Read the model definition and answer for the solid it produces. Units are mm, in the model's axes. Face numbers are marked on the shaded views. Coordinates: 2 decimals unless noted, no trailing zeros. Write each loop counter-clockwise with the first axis right and the second up, starting at its lowest first coordinate (ties: lowest second). Pieces come first, ordered by that corner, then holes. Notation, with made-up numbers: (26.25, 52.25) - (66.25, 52.25) arc R25 cw to (66.25, 77.25) - close; hole circle Ø1 at (-2.5, 59.25). An arc over 180 degrees is marked (long way). Return JSON: item names as keys, results as strings.
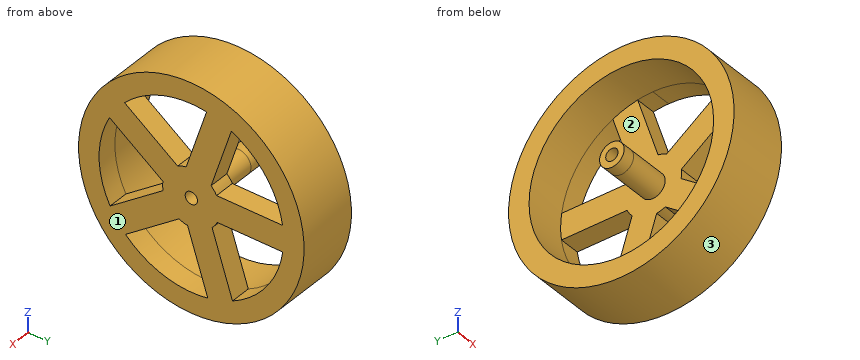
```python
from build123d import *

# Parameters (mm, degrees)
SKETCH1_R           = 27.5
BOSS_EXTRUDE1_DEPTH = 15
SKETCH2_R           = 1.5
CUT_EXTRUDE1_DEPTH  = 16
SKETCH3_R           = 22.5
SKETCH3_R_2         = 3
CUT_EXTRUDE2_DEPTH  = 10
SKETCH4_R           = 3
SKETCH4_R_2         = 1.5
BOSS_EXTRUDE2_DEPTH = 3
CUT_EXTRUDE3_DEPTH  = 6


with BuildPart() as part:
    # Sketch1 → Boss-Extrude1 (new body)
    with BuildSketch(Plane(origin=(0, 0, 0), x_dir=(0, 0, -1), z_dir=(1, 0, 0))):
        Circle(SKETCH1_R)
    extrude(amount=BOSS_EXTRUDE1_DEPTH)

    # Sketch2 → Cut-Extrude1 (cut, through all)
    with BuildSketch(Plane(origin=(15, 0, 0), x_dir=(0, 0, -1), z_dir=(1, 0, 0))):
        Circle(SKETCH2_R)
    extrude(amount=-CUT_EXTRUDE1_DEPTH, mode=Mode.SUBTRACT)

    # Sketch3 → Cut-Extrude2 (cut)
    with BuildSketch(Plane.ZY):
        Circle(SKETCH3_R)
        Circle(SKETCH3_R_2, mode=Mode.SUBTRACT)
    extrude(amount=-CUT_EXTRUDE2_DEPTH, mode=Mode.SUBTRACT)

    # Sketch4 → Boss-Extrude2 (add)
    with BuildSketch(Plane.ZY):
        Circle(SKETCH4_R)
        Circle(SKETCH4_R_2, mode=Mode.SUBTRACT)
    extrude(amount=BOSS_EXTRUDE2_DEPTH)

    # Sketch5 → Cut-Extrude3 (cut, through all)
    with BuildSketch(Plane.ZY.offset(-10)):
        with BuildLine():
            Line((5.074237821, 4.822044228), (20.272779151, 9.76034966))
            ThreePointArc((20.272779151, 9.76034966), (13.350301343, 18.111307353), (3.325036991, 22.252957759))
            Line((3.325036991, 22.252957759), (3.325036991, 6.1598806))
            ThreePointArc((3.325036991, 6.1598806), (4.252576382, 5.560179324), (5.074237821, 4.822044228))
        make_face()
        with BuildLine():
            Line((-3.018010865, 6.315980559), (-3.018010865, 22.296672631))
            ThreePointArc((-3.018010865, 22.296672631), (-13.099406882, 18.293592849), (-20.136327546, 10.03884022))
            Line((-20.136327546, 10.03884022), (-4.830901647, 5.065805886))
            ThreePointArc((-4.830901647, 5.065805886), (-3.973926406, 5.762630382), (-3.018010865, 6.315980559))
        make_face()
        with BuildLine():
            Line((-6.939471114, -0.91855357), (-22.138012444, 4.019751862))
            ThreePointArc((-22.138012444, 4.019751862), (-21.446180029, -6.805245196), (-15.769971823, -16.048613295))
            Line((-15.769971823, -16.048613295), (-6.310698406, -3.029040382))
            ThreePointArc((-6.310698406, -3.029040382), (-6.70859797, -1.998677884), (-6.939471114, -0.91855357))
        make_face()
        with BuildLine():
            Line((10.389948957, -19.957428709), (0.93067554, -6.937855796))
            ThreePointArc((0.93067554, -6.937855796), (-0.172215156, -6.997881246), (-1.270818148, -6.883677886))
            Line((-1.270818148, -6.883677886), (-10.664033269, -19.812329354))
            ThreePointArc((-10.664033269, -19.812329354), (-0.155061304, -22.499465682), (10.389948957, -19.957428709))
        make_face()
        with BuildLine():
            ThreePointArc((22.5, 0), (22.422695556, 1.863524623), (22.19131342, 3.714244025))
            Line((22.19131342, 3.714244025), (6.885887521, -1.258790309))
            ThreePointArc((6.885887521, -1.258790309), (6.60216315, -2.326250576), (6.154062305, -3.335793331))
            Line((6.154062305, -3.335793331), (15.547277427, -16.264444799))
            ThreePointArc((15.547277427, -16.264444799), (20.688931124, -8.844101365), (22.5, 0))
        make_face()
    extrude(amount=-CUT_EXTRUDE3_DEPTH, mode=Mode.SUBTRACT)


solid = part.part
```
(1) Straight lines are drawn through the part: line 1 (Y direction, x = 8.75, z = 0); line 2 (Y direction, x = 11, z = 0); line 3 (Y direction, x = -2.1, z = 0). For each, find the intervals that lie inside material, in ascending order. Write a range as from..to.
Answer:
{"line 1": "-27.5..-22.5, -3..-1.5, 1.5..3, 22.5..27.5", "line 2": "-27.5..-22.5, -7..-1.5, 1.5..27.5", "line 3": "-3..-1.5, 1.5..3"}
(2) A cutting plane is placed at A-A (z = 0). Determine the outline of the cut face in (x, y), and give its area (4 significant figures).
Answer:
{"outline": "(-3, -3) - (10, -3) - (10, -7) - (15, -7) - (15, -1.5) - (-3, -1.5) - close; (-3, 1.5) - (15, 1.5) - (15, 27.5) - (0, 27.5) - (0, 22.5) - (10, 22.5) - (10, 3) - (-3, 3) - close; (0, -27.5) - (15, -27.5) - (15, -22.5) - (0, -22.5) - close", "area": "321.5 mm²"}
(3) Flat-ended cylindrical pins translate along their axes: P1, Ø1, axis at x = 1, z = -9, coming from the +Y side; P2, Ø1.8, axis at y = 0, z = 0, coming from the +X side; P3, Ø12, axis at y = -11, z = 17, coming from the -X side; P4, Ø1.5, axis at x = 12, y = 10.5, coming from the +Z side. Find the tip coordinate at first contact, or state that the pin passes through.
Answer:
{"P1": "y = 26.15", "P2": "through", "P3": "x = 0", "P4": "z = 25.71"}
(4) Determine the mould class of the marked faces 1, 2 and 3 for opening direction Y: +Y half, -Y half, draft (parallel to the pull), parting line (faces both ways), or undercut.
Answer:
{"face 1": "draft", "face 2": "undercut", "face 3": "parting line"}
(5) A cutting plane is placed at D-D (y = 8.5). Determine the outline of the cut face in (x, z).
Answer:
{"outline": "(0, -26.15) - (15, -26.15) - (15, -15.4) - (10, -15.4) - (10, -20.83) - (0, -20.83) - close; (0, 20.83) - (10, 20.83) - (10, 16.39) - (15, 16.39) - (15, 26.15) - (0, 26.15) - close; (10, -3.02) - (15, -3.02) - (15, 3.33) - (10, 3.33) - close"}
(6) A cutting plane is placed at B-B (x = 6.75). Determine the outline of the cut face in (y, z), and give its area (3 significant figures).
Answer:
{"outline": "circle Ø55 at (0, 0); circle Ø6 at (0, 0); hole circle Ø45 at (0, 0); hole circle Ø3 at (0, 0)", "area": "807 mm²"}
(7) A cutting plane is placed at C-C (y = -11). Determine the outline of the cut face in (x, z), and give its area (3 significant figures).
Answer:
{"outline": "(0, -25.2) - (15, -25.2) - (15, -19.63) - (0, -19.63) - close; (0, 19.63) - (15, 19.63) - (15, 25.2) - (0, 25.2) - close; (10, -12.1) - (15, -12.1) - (15, -4.26) - (10, -4.26) - close; (10, 3.88) - (15, 3.88) - (15, 11.72) - (10, 11.72) - close", "area": "246 mm²"}
